```python
from build123d import *

# Parameters (mm, degrees)
EXTRUDE_1_DEPTH     = 85
FILLET_1_R          = 0.8
SKETCH_2_R          = 2
CUT_EXTRUDE_1_DEPTH = 2
SKETCH_3_R          = 2
CUT_EXTRUDE_2_DEPTH = 400


with BuildPart() as part:
    # 草图1 → 凸台-拉伸1 (new body)
    with BuildSketch(Plane.XY):
        Polygon((0, 0), (0, 15), (-2, 15), (-2, 2), (-15, 2), (-15, 0), align=None)
    extrude(amount=EXTRUDE_1_DEPTH)

    # 圆角1
    fillet_1_edges = [part.edges().sort_by_distance(p)[0] for p in [
        (-15, 2, 42.5),
        (-2, 15, 42.5),
    ]]
    fillet(fillet_1_edges, radius=FILLET_1_R)

    # 草图2 → 切除-拉伸1 (cut)
    with BuildSketch(Plane(origin=(0, 2, 0), x_dir=(1, 0, 0), z_dir=(0, 1, 0))):
        with Locations((-8, -15)):
            Circle(SKETCH_2_R)
    extrude(amount=-CUT_EXTRUDE_1_DEPTH, mode=Mode.SUBTRACT)

    # 草图3 → 切除-拉伸2 (cut)
    with BuildSketch(Plane.ZY.offset(2)):
        with Locations((75, 9)):
            Circle(SKETCH_3_R)
    extrude(amount=-CUT_EXTRUDE_2_DEPTH, mode=Mode.SUBTRACT)


solid = part.part
```
The model under review builds one solid part; all positions refer to its coordinate system, in mm. A direction names the side the tool comes from. Coordinates: 2 decimals unless noted, no trailing zeros. Order: outer loops, then holes, each group sorted by start corner. A loop starts at its lowest first (then second) coordinate and runs counter-clockwise, first axis right, second up. Notation, with made-up numbers: (71.25, 17) -> (102.25, 17) arc R12 cw to (102.25, 33) -> close; hole circle Ø9 at (66, -15). An arc over 180 degrees is marked (long way). Answer in a Markdown table with one row per item. Add a question column.
Item 1: Mouldability with a two-part tool opening along Z and no side actions: class faces 1 (the cylindrical face through (-1.014, 9.601, 76.908)), 2 (the flat face through (-8, 0, 42)) as +Z half, -Z half, draft (parallel to the pull), parting line (faces both ways), or undercut.
Item 2: We need section B-B on z = 75. Write out the cut boundary in (x, y), plus the area to 3 significant figures.
Item 3: We need section A-A on y = 9. Write out the cut boundary in (x, z).
Item 4: We need section D-D on z = 49. Write out the cut boundary in (x, y).
Item 5: Machinability: for faces 3 (the cylindrical face through (-8, 1, 13)), 4 (the flat face through (-8, 2, 42)), which of the approach directions +Z, -Z, +X, -X, +Y, -Y give a long, thin tool a straight path to every point of the face, cutting with its end or side? Answer none if there is none.
Item 6: Clearance check with a flat-ended pin moving along its axis: pin 1 (6 mm diameter, centred on x = -9.5, z = 25.5, fed in from +Y). State where the tip first meets the part, or that it passes through.
Item 7: To check wall thickness, follow probe 1 along X at (y, z) = (1.3, 15); probe 2 along Z at (x, y) = (-8, 0.55); probe 3 along Y at (x, z) = (-0.4, 75). State the ranges of each line that lie inside material, in increasing order.
Item 8: We need section C-C on x = -8. Write out the cut boundary in (y, z).
Final values:
| question | item | result |
|---|---|---|
| 1 | face 1 | undercut |
| 1 | face 2 | draft |
| 2 | outline | (-15, 0) -> (0, 0) -> (0, 7) -> (-2, 7) -> (-2, 2) -> (-14.2, 2) arc R0.8 ccw to (-15, 1.2) -> close; (-2, 11) -> (0, 11) -> (0, 15) -> (-1.2, 15) arc R0.8 ccw to (-2, 14.2) -> close |
| 2 | area | 47.7 mm2 |
| 3 | outline | (-2, 0) -> (0, 0) -> (0, 73) -> (-2, 73) -> close; (-2, 77) -> (0, 77) -> (0, 85) -> (-2, 85) -> close |
| 4 | outline | (-15, 0) -> (0, 0) -> (0, 15) -> (-1.2, 15) arc R0.8 ccw to (-2, 14.2) -> (-2, 2) -> (-14.2, 2) arc R0.8 ccw to (-15, 1.2) -> close |
| 5 | face 3 | +Y, -Y |
| 5 | face 4 | +Z, -Z, -X, +Y |
| 6 | pin 1 | stops at y = 2 |
| 7 | probe 1 | x = -14.99 to -10, -6 to 0 |
| 7 | probe 2 | z = 0 to 13, 17 to 85 |
| 7 | probe 3 | y = 0 to 7, 11 to 15 |
| 8 | outline | (0, 0) -> (2, 0) -> (2, 13) -> (0, 13) -> close; (0, 17) -> (2, 17) -> (2, 85) -> (0, 85) -> close |
